```python
from build123d import *

# Parameters (mm, degrees)
SKETCH1_R           = 2.4999999999999987
SKETCH1_R_2         = 2.4999999999999996
SKETCH1_R_3         = 2.4999999988368367
BOSS_EXTRUDE1_DEPTH = 1.5


with BuildPart() as part:
    # Sketch1 → Boss-Extrude1 (new, symmetric)
    with BuildSketch(Plane(origin=(0, 0, 0), x_dir=(1, 0, 0), z_dir=(0, 1, 0))):
        with BuildLine():
            Line((-41.79617581077867, 2.382798182125341), (-37.73330547981784, 3.726907894077695))
            ThreePointArc((-37.73330547981784, 3.726907894077695), (-33.34023665036322, 4.48261370370704), (-28.919065231416493, 3.9139413064841877))
            Line((-28.919065231416493, 3.9139413064841877), (-27.228879505558364, 3.4332944614597887))
            ThreePointArc((-27.228879505558364, 3.4332944614597887), (-23.456808752947794, 2.864896052239951), (-19.663338722278937, 3.26636789523878))
            Line((-19.663338722278937, 3.26636789523878), (-11.919945267506879, 5.103463979240285))
            ThreePointArc((-11.919945267506879, 5.103463979240285), (-9.469729211186351, 5.474383326712289), (-6.991881476316525, 5.436826865477882))
            Line((-6.991881476316525, 5.436826865477882), (5.951872192796172, 4.166165679329836))
            ThreePointArc((5.951872192796172, 4.166165679329836), (8.429719927543827, 4.128609218087167), (10.879935983748245, 4.499528565510892))
            Line((10.879935983748245, 4.499528565510892), (21.40551753025073, 6.996690146393965))
            ThreePointArc((21.40551753025073, 6.996690146393965), (24.83264502259487, 7.401769909560215), (28.261649532088523, 7.012899060487261))
            Line((28.261649532088523, 7.012899060487261), (35.99495155066682, 5.216777544396412))
            ThreePointArc((35.99495155066682, 5.216777544396412), (39.42395606023976, 4.82790669529539), (42.85108355268613, 5.232986458392139))
            Line((42.85108355268613, 5.232986458392139), (49.96600006451842, 6.920978336659753))
            ThreePointArc((49.96600006451842, 6.920978336659753), (53.72001531855511, 7.32326878816774), (57.455567828585835, 6.77544073145873))
            Line((57.455567828585835, 6.77544073145873), (66.18925821321116, 4.3413933248153))
            ThreePointArc((66.18925821321116, 4.3413933248153), (67.36926268792493, 4.088133405140102), (68.57118312482231, 3.9788703710124524))
            ThreePointArc((68.57118312482231, 3.9788703710124524), (76.70834195009273, 3.69798054493333), (84.84283443476778, 3.3482880245078643))
            ThreePointArc((84.84283443476778, 3.3482880245078643), (90.6755684371097, 4.07235098588054), (96.32527960365518, 5.692788225862035))
            Line((96.32527960365518, 5.692788225862035), (103.59933222252589, 9.439170279671533))
            ThreePointArc((103.59933222252589, 9.439170279671533), (108.01760653283236, 11.089221722684941), (112.69942544373606, 11.658773591445987))
            ThreePointArc((112.69942544373606, 11.658773591445987), (137.42059205461962, -12.991414338135115), (112.69942544373606, -37.64160226771621))
            ThreePointArc((112.69942544373606, -37.64160226771621), (108.01760653283236, -37.07205039895516), (103.59933222252589, -35.42199895594175))
            Line((103.59933222252589, -35.42199895594175), (96.32527960365518, -31.675616902132255))
            ThreePointArc((96.32527960365518, -31.675616902132255), (88.5441551766424, -27.463864954095598), (79.9703022290949, -25.278962792836175))
            ThreePointArc((79.9703022290949, -25.278962792836175), (-3.2675277579170765, -27.22969716665807), (-86.51046185027334, -25.510502808965498))
            ThreePointArc((-86.51046185027334, -25.510502808965498), (-94.72463382860796, -23.967931939620144), (-102.76843470025015, -21.698699973958888))
            ThreePointArc((-102.76843470025015, -21.698699973958888), (-113.75910937557403, -17.35916690176714), (-124.45852861685042, -12.344298508393459))
            ThreePointArc((-124.45852861685042, -12.344298508393459), (-133.23144555995484, 4.202899533030633), (-120.59919444516926, 18.030410751095733))
            ThreePointArc((-120.59919444516926, 18.030410751095733), (-86.83004932052131, 27.105129355217315), (-51.97527685246112, 29.907006653257785))
            ThreePointArc((-51.97527685246112, 29.907006653257785), (-47.10250450667497, 27.022733824765), (-51.95035427562549, 24.096765147433302))
            ThreePointArc((-51.95035427562549, 24.096765147433302), (-84.17625346987383, 21.176955554132093), (-114.64829350025539, 10.291706667413088))
            ThreePointArc((-114.64829350025539, 10.291706667413088), (-117.36336095050851, 5.634125667179891), (-114.23380520696547, 1.244304158141715))
            ThreePointArc((-114.23380520696547, 1.244304158141715), (-84.82863856721416, -4.964735101077579), (-55.03457582625992, -1.023945964096185))
            ThreePointArc((-55.03457582625992, -1.023945964096185), (-52.956149124988286, 1.029337853892025), (-53.43468142437476, 3.9114965636467445))
            ThreePointArc((-53.43468142437476, 3.9114965636467445), (-53.00487930043318, 4.054737535668091), (-52.611913679317254, 3.829291616670397))
            ThreePointArc((-52.611913679317254, 3.829291616670397), (-51.09811473462323, 3.897658149961778), (-49.58701407449473, 4.010954322846273))
            ThreePointArc((-49.58701407449473, 4.010954322846273), (-45.88836824044927, 2.255302591622458), (-41.79617581077867, 2.382798182125341))
        make_face()
        with Locations(Location((-27.228879503846553, -2.927214905609624, 0), (0, 0, 270))):
            Circle(SKETCH1_R, mode=Mode.SUBTRACT)
        with Locations(Location((10.879935983748245, -22.16932690789429, 0), (0, 0, 270))):
            Circle(SKETCH1_R_2, mode=Mode.SUBTRACT)
        with Locations(Location((53.72001531851656, 1.3232687879424379, 0), (0, 0, 270))):
            Circle(SKETCH1_R_3, mode=Mode.SUBTRACT)
        with BuildLine():
            Line((-7.347962122783413, -8.651271752579847), (32.25203787721659, -4.6713220041533745))
            ThreePointArc((32.25203787721659, -4.6713220041533745), (37.73209037371569, -9.200078584871521), (33.1443469248767, -14.630844790428428))
            Line((33.1443469248767, -14.630844790428428), (-7.346014603537373, -10.64144043499709))
            ThreePointArc((-7.346014603537373, -10.64144043499709), (-8.24796164398419, -9.647237759156878), (-7.347962122783413, -8.651271752579847))
        make_face(mode=Mode.SUBTRACT)
        with BuildLine():
            Line((86.87503313674924, -2.91833741505861), (107.18489994547878, 4.935508738787573))
            ThreePointArc((107.18489994547878, 4.935508738787573), (110.24885192022663, 5.593844362539373), (113.36611131404287, 5.271507010179491))
            ThreePointArc((113.36611131404287, 5.271507010179491), (123.48655350207885, -1.4751872230410612), (127.40034273906164, -12.991414338135112))
            ThreePointArc((127.40034273906164, -12.991414338135112), (123.48655350207883, -24.507641453229162), (113.36611131404287, -31.25433568644971))
            ThreePointArc((113.36611131404287, -31.25433568644971), (110.24885192022663, -31.576673038809595), (107.18489994547878, -30.9183374150578))
            Line((107.18489994547878, -30.9183374150578), (86.87503313674924, -23.064491261211614))
            ThreePointArc((86.87503313674924, -23.064491261211614), (81.86219058303507, -19.097603567215177), (79.9703022290949, -12.991414338135112))
            ThreePointArc((79.9703022290949, -12.991414338135112), (81.86219058303507, -6.8852251090550425), (86.87503313674924, -2.91833741505861))
        make_face(mode=Mode.SUBTRACT)
    extrude(amount=BOSS_EXTRUDE1_DEPTH, both=True)


solid = part.part
```
Can you work these out from the model? Positions are in its coordinate system, mm. A direction names the side the tool comes from. Coordinates: 2 decimals unless noted, no trailing zeros. Loops run counter-clockwise (first coordinate to the right, second up) from the corner with the lowest first, then second, coordinate; pieces in that order, holes last. Notation, with made-up numbers: (85.25, 51) -> (93.25, 51) arc R25 ccw to (93.25, 74) -> close; hole circle Ø6 at (89.5, -37.5). An arc over 180 degrees is marked (long way). Answer as a JSON object with one key per item and string values.
1) Imagine slicing it at B-B (x = 99). Please give me the cut outline in (y, z).
Results:
{"outline": "(-1.5, -7.07) -> (1.5, -7.07) -> (1.5, -1.77) -> (-1.5, -1.77) -> close; (-1.5, 27.75) -> (1.5, 27.75) -> (1.5, 33.05) -> (-1.5, 33.05) -> close"}
2) For faces 1 (the face through (88.66, 0.02, 27.51)), 2 (the face through (96.888, 0.021, -0.954)), 3 (the face through (4, 1.5, 3)), which set-ups out of +Z, -Z, +X, -X, +Y, -Y let a thin tool reach every point of the face, with its end or its side?
Results:
{"face 1": "+Z, +Y, -Y", "face 2": "+Y, -Y", "face 3": "+Z, -Z, +X, -X, +Y"}
3) For P1, Ø1.5, axis at x = -3.5, y = 0.5, coming from the +Z side; P2, Ø1, axis at y = 0.5, z = 30, coming from the +X side; P3, Ø4, axis at x = 10.88, z = 22.17, coming from the -Y side, each with a flat end and sliding along its axis, tell me the tip position at first contact or that it passes through.
Results:
{"P1": "stops at z = 27.23", "P2": "stops at x = 131.08", "P3": "passes through"}
4) Thinking about a two-plate mould opening in X: for faces 4 (the face through (97.172, 0.021, 27.046)), 5 (the face through (79.97, -0.02, 13.17)), 6 (the face through (4, -1.5, 3)), 7 (the face through (-133.264, 0.021, -3.925)), which applies, pulls with the +X half, pulls with the -X half, needs draft (parallel to the pull), parting line crosses it, or undercut?
Results:
{"face 4": "undercut", "face 5": "undercut", "face 6": "needs draft", "face 7": "pulls with the -X half"}
5) Imagine slicing it at A-A (x = -82). Please give me the cut outline in (y, z).
Results:
{"outline": "(-1.5, -27.88) -> (1.5, -27.88) -> (1.5, -21.64) -> (-1.5, -21.64) -> close; (-1.5, 5.03) -> (1.5, 5.03) -> (1.5, 25.7) -> (-1.5, 25.7) -> close"}
6) If I drill on line 1 (Z direction, x = -56.5, y = -1.2); line 2 (Z direction, x = 30.5, y = -0.3); line 3 (X direction, y = 1.3, z = 17), over which ranges is the centre line in solid material (lowest first)?
Results:
{"line 1": "z = -29.9 to -24.18, 1.47 to 26.55", "line 2": "z = -6.49 to 4.85, 14.37 to 26.88", "line 3": "x = -114.59 to 80.74, 126.97 to 137.09"}
7) Imagine slicing it at D-D (z = -15). Please give me the cut outline in (x, y), then the cut area to 3 significant figures.
Results:
{"outline": "(-127.07, -1.5) -> (-104.24, -1.5) -> (-104.24, 1.5) -> (-127.07, 1.5) -> close", "area": "68.5 mm^2"}
8) Imagine slicing it at C-C (y = -0.8). Count the separate pieces of the cut face and the enclosed holes in it, then the cut area to 3 significant figures.
Results:
{"separate pieces": "1", "enclosed holes": "5", "area": "7,040 mm^2"}
